The figure shows three views and two pictorial views of one solid part (mm, origin at its lowest corner). Answer the questions. A direction names the side the tool comes from. Coordinates: 2 decimals unless noted, no trailing zeros. Order: outer loops, then holes, each group sorted by start corner. A loop starts at its lowest first (then second) coordinate and runs counter-clockwise, first axis right, second up. Notation, with made-up numbers: M 46.25,-7 L 66.25,-7 A19 ccw 66.25,29 Z; hole C 18.5,-30.75 d7. An arc over 180 degrees is marked long. Use a Markdown table: item, result.
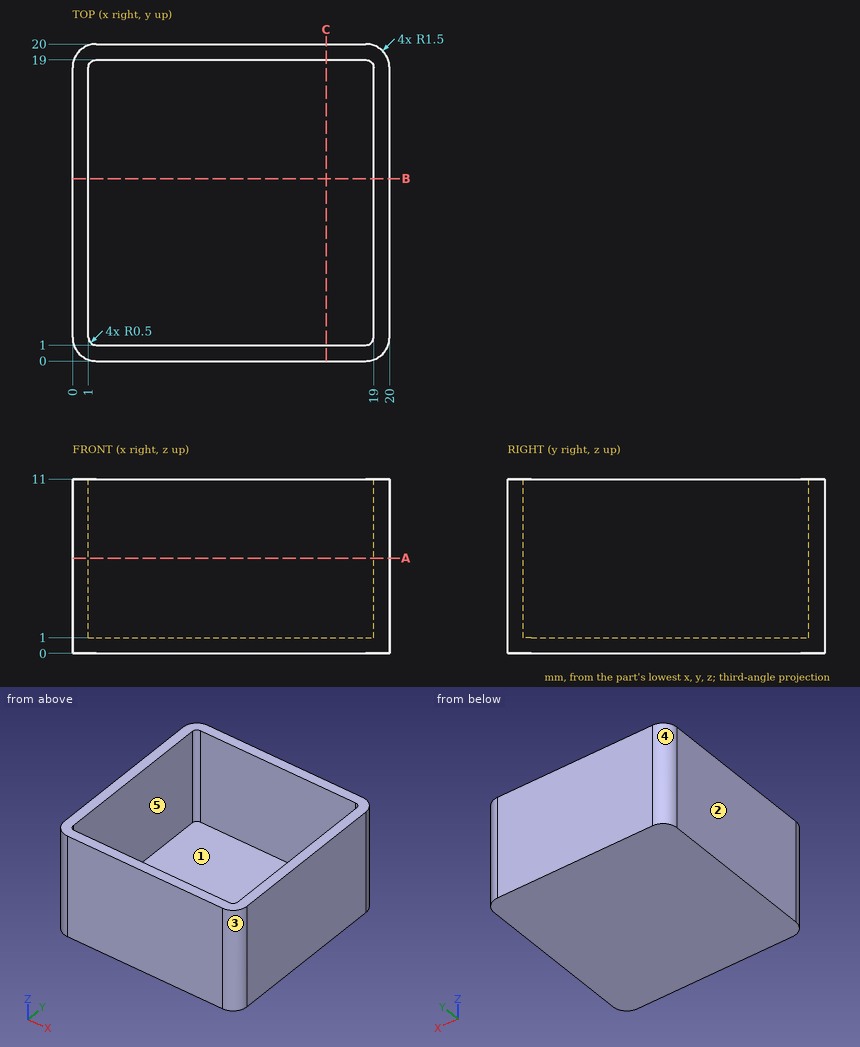
1. For a pull along Y with two mould halves and no side action, classify the marked faces 3, 4 and 5 as +Y half, -Y half, draft (parallel to the pull), parting line (faces both ways), or undercut.
Answers below:
| item | result |
|---|---|
| face 3 | -Y half |
| face 4 | +Y half |
| face 5 | undercut |
2. Flat-ended cylindrical pins translate along their axes: P1, Ø1, axis at x = 15.5, y = 10.5, coming from the -Z side; P2, Ø9, axis at x = 10.5, y = 12.5, coming from the +Z side. Find the tip coordinate at first contact, or state that the pin passes through.
Answers below:
| item | result |
|---|---|
| P1 | z = 0 |
| P2 | z = 1 |
3. Find the intervals of material crossed by probe 1 along Y at (x, z) = (17.5, 6.25); probe 2 along Z at (x, y) = (5.5, 5.25), in increasing order.
Answers below:
| item | result |
|---|---|
| probe 1 | 0 to 1, 19 to 20 |
| probe 2 | 0 to 1 |
4. Section B-B on y = 11.5 is taken. Determine the outline of the cut face in (x, z), then the cut area to 3 significant figures.
Answers below:
| item | result |
|---|---|
| outline | M 0,0 L 20,0 L 20,11 L 19,11 L 19,1 L 1,1 L 1,11 L 0,11 Z |
| area | 40.0 mm² |
5. Section A-A on z = 6 is taken. Determine the outline of the cut face in (x, y), then the cut area to 3 significant figures.
Answers below:
| item | result |
|---|---|
| outline | M 0,1.5 A1.5 ccw 1.5,0 L 18.5,0 A1.5 ccw 20,1.5 L 20,18.5 A1.5 ccw 18.5,20 L 1.5,20 A1.5 ccw 0,18.5 Z; hole M 1,1.5 A0.5 ccw 1.5,1 L 18.5,1 A0.5 ccw 19,1.5 L 19,18.5 A0.5 ccw 18.5,19 L 1.5,19 A0.5 ccw 1,18.5 Z |
| area | 74.3 mm² |
6. For the marked faces 1 and 2, determine the directions among +Z, -Z, +X, -X, +Y, -Y from which every point of the face is accessible in a straight line to the end or side of a thin tool.
Answers below:
| item | result |
|---|---|
| face 1 | +Z |
| face 2 | +Z, -Z, -X, +Y, -Y |
